CAD build for the part. Positions are in the model's coordinates, mm. A direction names the side the tool comes from. Round coordinates to 2 decimals unless told otherwise and drop trailing zeros. Order: outer loops, then holes, each group sorted by start corner. A loop starts at its lowest first (then second) coordinate and runs counter-clockwise, first axis right, second up. Notation, with made-up numbers: (54, -8) - (112, -8) arc R23 cw to (112, 16) - close; hole circle Ø1 at (28, -17.5). An arc over 180 degrees is marked (long way). Write item = value, one per line.
Autodesk Inventor part; units mm, degrees
ref_plane "YZ Plane" through (0, 0, 0) normal (1, 0, 0) x (0, 1, 0)
ref_plane "XZ Plane" through (0, 0, 0) normal (0, 1, 0) x (-1, 0, 0)
ref_plane "XY Plane" through (0, 0, 0) normal (0, 0, 1) x (1, 0, 0)
sketch "Sketch1" plane through (0, 0, 0) normal (0, 1, 0) x (-1, 0, 0)
  arc A0 (139.7, 0) -> (-139.7, 0) centre (0, 0) ccw
  arc A1 (142.875, 0) -> (-142.875, 0) centre (0, 0) ccw
  line L0 (139.7, 0) -> (142.875, 0)
  line L1 (-139.7, 0) -> (-142.875, 0)
  dimension "d0" = 279.4
  dimension "d1" = 3.175
extrude "Extrusion1" add sketch "Sketch1" along normal blind 57.15
sketch "Sketch2" plane through (0, 57.15, 0) normal (0, 1, 0) x (1, 0, 0)
  arc A0 (-88.9, 0) -> (88.9, 0) centre (0, 0) ccw
  arc A1 (-142.875, 0) -> (142.875, 0) centre (0, 0) ccw
  line L0 (-139.7, 0) -> (-142.875, 0)
  line L1 (-142.875, 0) -> (-88.9, 0)
  line L2 (88.9, 0) -> (142.875, 0)
  dimension "d4" = 177.8
extrude "Extrusion2" add sketch "Sketch2" along normal blind 3.175
sketch "Sketch3" plane through (0, 0, 0) normal (0, -1, 0) x (1, 0, 0)
  arc A0 (142.875, 0) -> (-142.875, 0) centre (0, 0) ccw
  arc A1 (88.9, 0) -> (-88.9, 0) centre (0, 0) ccw
  line L0 (-139.7, 0) -> (-88.9, 0)
  line L1 (88.9, 0) -> (139.7, 0)
  line L2 (139.7, 0) -> (142.875, 0)
  line L3 (-142.875, 0) -> (-139.7, 0)
extrude "Extrusion3" add sketch "Sketch3" along normal blind 3.175
sketch "Sketch4" plane through (0, 60.325, 0) normal (0, 1, 0) x (1, 0, 0)
  line L0 (-88.9, 0) -> (-142.875, 0)
  line L1 (142.875, 0) -> (88.9, 0)
  point P0 (0, 0)
properties part number "Holster"
(1) Drop flat-ended pins along their axis: pin 1 (10 mm diameter, centred on y = 28.5, z = 66, fed in from -X); pin 2 (3 mm diameter, centred on y = 42, z = 76, fed in from +X); pin 3 (1.5 mm diameter, centred on x = -31, y = 12, fed in from -Z). Give the stop position or say it passes through.
Solved:
pin_1 = -129.2
pin_2 = 121.91
pin_3 = 136.04
(2) Band-saw the part on C-C on z = 106.5. List the corners of the cut face in (x, y) (3 decimals).
Solved:
outline = (-95.242, -3.175) - (95.242, -3.175) - (95.242, 60.325) - (-95.242, 60.325) - close; hole (-90.409, 0) - (90.409, 0) - (90.409, 57.15) - (-90.409, 57.15) - close
(3) Band-saw the part on B-B on x = 0. List the corners of the cut face in (y, z) (3 decimals), plus the area to 3 significant figures.
Solved:
outline = (-3.175, 88.9) - (0, 88.9) - (0, 139.7) - (57.15, 139.7) - (57.15, 88.9) - (60.325, 88.9) - (60.325, 142.875) - (-3.175, 142.875) - close
area = 524 mm²
(4) Probe line 1 along Y through (x, z) = (87, 81.5) (3 decimals); line 2 along X through (y, z) = (22, 14); line 3 along X through (y, z) = (34, 53.5). List the from-to ranges inside material, lowest first.
Solved:
line_1 = -3.175 to 0, 57.15 to 60.325
line_2 = -142.19 to -139, 139 to 142.19
line_3 = -132.48 to -129.05, 129.05 to 132.48
(5) Pull direction Y, two halves, no side cores. Call faces 3 (the flat face through (140, 29, 0)), 4 (the flat face through (-2, 60.325, 102)), 5 (the flat face through (-2, -3.175, 104)), 6 (the cylindrical face through (3.072, 28.175, 139.666)): released by +Y, released by -Y, zero draft, split by the parting line, or undercut.
Solved:
face_3 = zero draft
face_4 = released by +Y
face_5 = released by -Y
face_6 = undercut
(6) Band-saw the part on D-D on y = 19.5. List the corners of the cut face in (x, z) (3 decimals), plus the area to 3 significant figures.
Solved:
outline = (-142.875, 0) - (-139.7, 0) arc R139.7 cw to (139.7, 0) - (142.875, 0) arc R142.875 ccw to start
area = 1,410 mm²
(7) Tool access for faces 1 (the cylindrical face through (-1.95, -1.57, 88.88)), 2 (the flat face through (-2, 0, 102)): list every direction of +Z, -Z, +X, -X, +Y, -Y with a clear straight run to the whole face (end or side of a thin tool).
Solved:
face_1 = -Z, +Y, -Y
face_2 = -Z
(8) Band-saw the part on A-A on z = 26. List the corners of the cut face in (x, y) (3 decimals).
Solved:
outline = (-140.489, -3.175) - (-85.013, -3.175) - (-85.013, 0) - (-137.259, 0) - (-137.259, 57.15) - (-85.013, 57.15) - (-85.013, 60.325) - (-140.489, 60.325) - close; (85.013, -3.175) - (140.489, -3.175) - (140.489, 60.325) - (85.013, 60.325) - (85.013, 57.15) - (137.259, 57.15) - (137.259, 0) - (85.013, 0) - close
